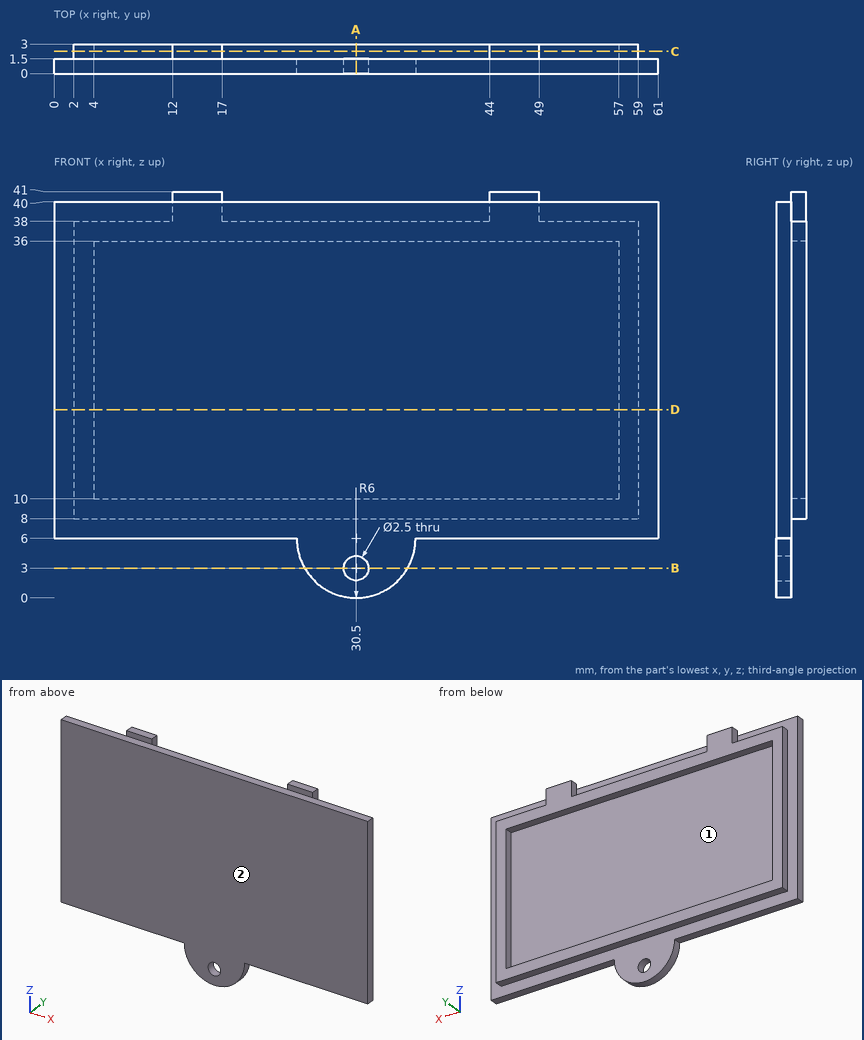
Study the drawing (mm; zero at the part's minimum x, y, z) and answer. Coordinates: 2 decimals unless noted, no trailing zeros. Write each loop counter-clockwise with the first axis right and the second up, starting at its lowest first coordinate (ties: lowest second). Pieces come first, ordered by that corner, then holes.
Q1. Each of these flat-tipped pins is pushed along its axis until it touches: pin 1 Ø1.5 at (y, z) = (2.5, 31) entering from -X; pin 2 Ø12 at (x, z) = (30, 23.5) entering from +Y; pin 3 Ø0.8 at (y, z) = (2, 39.5) entering from +X. Where does it stop, or does it pass through?
Q2. A cutting plane is placed at D-D, the plane z = 19. Give the vertices of the cut face in (x, y), then the cut area to 3 significant figures.
Q3. A cutting plane is placed at A-A, the plane x = 30.5. Give the vertices of the cut face in (y, z).
Q4. Find the intervals of material crossed by line 1 (Z direction, x = 47.5, y = 2.3); line 2 (X direction, y = 1.6, z = 32.5); line 3 (Z direction, x = 52.5, y = 0.5), in increasing order.
Q5. A cutting plane is placed at C-C, the plane y = 2.25. Give the vertices of the cut face in (x, z).
Q6. A cutting plane is placed at B-B, the plane z = 3. Give the vertices of the cut face in (x, y).
Q7. Determine the mould class of the marked faces 1 and 2 for opening direction Z: released by +Z, released by -Z, zero draft, split by the parting line, or undercut.
Findings below:
1. pin 1: stops at x = 2
1. pin 2: stops at y = 1.5
1. pin 3: stops at x = 49
2. outline: (0, 0) - (61, 0) - (61, 1.5) - (59, 1.5) - (59, 3) - (57, 3) - (57, 1.5) - (4, 1.5) - (4, 3) - (2, 3) - (2, 1.5) - (0, 1.5) - close
2. area: 97.5 mm2
3. outline: (0, 0) - (1.5, 0) - (1.5, 1.75) - (0, 1.75) - close; (0, 4.25) - (1.5, 4.25) - (1.5, 8) - (3, 8) - (3, 10) - (1.5, 10) - (1.5, 36) - (3, 36) - (3, 38) - (1.5, 38) - (1.5, 40) - (0, 40) - close
4. line 1: z = 8 to 10, 36 to 41
4. line 2: x = 2 to 4, 57 to 59
4. line 3: z = 6 to 40
5. outline: (2, 8) - (59, 8) - (59, 38) - (49, 38) - (49, 41) - (44, 41) - (44, 38) - (17, 38) - (17, 41) - (12, 41) - (12, 38) - (2, 38) - close; hole (4, 10) - (57, 10) - (57, 36) - (4, 36) - close
6. outline: (25.3, 0) - (29.25, 0) - (29.25, 1.5) - (25.3, 1.5) - close; (31.75, 0) - (35.7, 0) - (35.7, 1.5) - (31.75, 1.5) - close
7. face 1: undercut
7. face 2: zero draft
